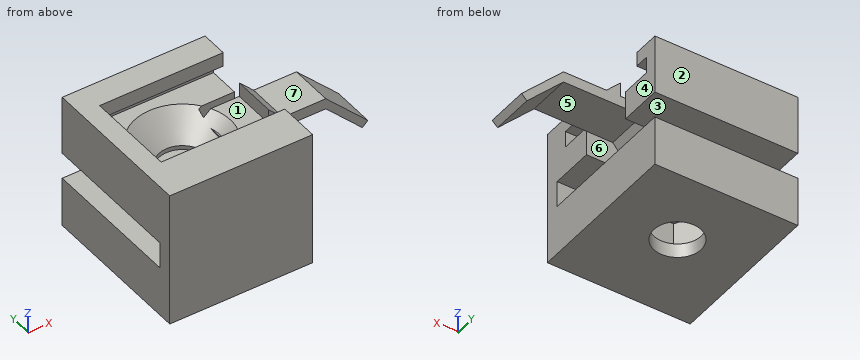
```python
from build123d import *

# Parameters (mm, degrees)
CROQUIS1_W               = 20
CROQUIS1_H               = 20
CROQUIS1_R               = 3.1
SALIENTE_EXTRUIR1_DEPTH  = 4
SALIENTE_EXTRUIR2_DEPTH  = 2.3
SALIENTE_EXTRUIR4_DEPTH  = 2
SALIENTE_EXTRUIR5_DEPTH  = 4
SALIENTE_EXTRUIR6_START  = -6
SALIENTE_EXTRUIR6_DEPTH  = 6
CROQUIS10_W              = 5
CROQUIS10_H              = 1
CORTAR_EXTRUIR2_DEPTH    = 4
CORTAR_EXTRUIR3_START    = -13
CROQUIS11_W              = 2.5
CROQUIS11_H              = 6
CORTAR_EXTRUIR3_DEPTH    = 13
SALIENTE_EXTRUIR7_START  = -6
SALIENTE_EXTRUIR7_DEPTH  = 6
CROQUIS14_W              = 20
CROQUIS14_H              = 19
SALIENTE_EXTRUIR8_DEPTH  = 2
CROQUIS15_W              = 20
CROQUIS15_H              = 7
SALIENTE_EXTRUIR9_DEPTH  = 20
CORTAR_EXTRUIR4_DEPTH    = 5
CROQUIS17_R              = 3.3
CORTAR_EXTRUIR5_DEPTH    = 2
SALIENTE_EXTRUIR10_START = -6
SALIENTE_EXTRUIR10_DEPTH = 6


with BuildPart() as part:
    # Croquis1 → Saliente-Extruir1 (new body)
    with BuildSketch(Plane.XY):
        Rectangle(CROQUIS1_W, CROQUIS1_H)
        Circle(CROQUIS1_R, mode=Mode.SUBTRACT)
    extrude(amount=SALIENTE_EXTRUIR1_DEPTH)

    # Croquis3 → Saliente-Extruir2 (add)
    with BuildSketch(Plane.XY.offset(4)):
        Polygon((10, 10), (-10, 10), (-10, -10), (10, -10), (10, -8.3), (-7.3, -8.3), (-7.3, 8.3), (10, 8.3), align=None)
    extrude(amount=SALIENTE_EXTRUIR2_DEPTH)

    # Croquis6 → Saliente-Extruir4 (add)
    with BuildSketch(Plane.XY.offset(6.3)):
        Polygon((10, 10), (10, 6.3), (-7.3, 6.3), (-7.3, -6.3), (10, -6.3), (10, -10), (-10, -10), (-10, 10), align=None)
    extrude(amount=SALIENTE_EXTRUIR4_DEPTH)

    # Croquis7 → Saliente-Extruir5 (add)
    with BuildSketch(Plane.XY.offset(4)):
        Polygon((10, 0), (10, 3), (18, 3), (18, 0), (18, -3), (10, -3), align=None)
    extrude(amount=-SALIENTE_EXTRUIR5_DEPTH)

    # Croquis9 → Saliente-Extruir6 (add)
    with BuildSketch(Plane.XZ.offset(3).offset(SALIENTE_EXTRUIR6_START)):
        Polygon((12, 4), (10, 6), (10, 4), align=None)
    extrude(amount=SALIENTE_EXTRUIR6_DEPTH)

    # Croquis10 → Cortar-Extruir2 (cut)
    with BuildSketch(Plane.XY.offset(4)):
        with Locations((7.5, 3.5)):
            Rectangle(CROQUIS10_W, CROQUIS10_H)
        with Locations((7.5, -3.5)):
            Rectangle(CROQUIS10_W, CROQUIS10_H)
    extrude(amount=-CORTAR_EXTRUIR2_DEPTH, mode=Mode.SUBTRACT)

    # Croquis11 → Cortar-Extruir3 (cut)
    with BuildSketch(Plane(origin=(18, 0, 0), x_dir=(0, 0, -1), z_dir=(1, 0, 0)).offset(CORTAR_EXTRUIR3_START)):
        with Locations((-1.25, 0)):
            Rectangle(CROQUIS11_W, CROQUIS11_H)
    extrude(amount=CORTAR_EXTRUIR3_DEPTH, mode=Mode.SUBTRACT)

    # Croquis12 → Saliente-Extruir7 (add)
    with BuildSketch(Plane(origin=(0, 3, 0), x_dir=(1, 0, 0), z_dir=(0, 1, 0)).offset(SALIENTE_EXTRUIR7_START)):
        Polygon((18, -2.5), (23.125934171, 2.625934171), (23.875934171, 1.875934171), (18, -4), align=None)
    extrude(amount=SALIENTE_EXTRUIR7_DEPTH)

    # Croquis13 → Refrentado para tornillo tapón con cabeza plana de clavija de M61 (revolve, cut)
    with BuildSketch(Plane(origin=(0, 0, 4), x_dir=(0, -1, 0), z_dir=(1, 0, 0))):
        Polygon((0, 0), (0, 6.625934171), (3.3, 6.625934171), (3.3, 3.42), (6.72, 0), align=None)
    revolve(axis=Axis((0, 0, 10.35), (0, 0, -1)), mode=Mode.SUBTRACT)

    # Croquis14 → Saliente-Extruir8 (add)
    with BuildSketch(Plane.XZ.offset(10)):
        with Locations((0, -1.2)):
            Rectangle(CROQUIS14_W, CROQUIS14_H)
    extrude(amount=SALIENTE_EXTRUIR8_DEPTH)

    # Croquis15 → Saliente-Extruir9 (add)
    with BuildSketch(Plane(origin=(0, -10, 0), x_dir=(1, 0, 0), z_dir=(0, 1, 0))):
        with Locations((0, 7.2)):
            Rectangle(CROQUIS15_W, CROQUIS15_H)
    extrude(amount=SALIENTE_EXTRUIR9_DEPTH)

    # Croquis16 → Cortar-Extruir4 (cut)
    with BuildSketch(Plane.XY.offset(-3.7)):
        Polygon((5.802370205, 0), (2.901185103, 5.025), (-2.901185103, 5.025), (-5.802370205, 0), (-2.901185103, -5.025), (2.901185103, -5.025), align=None)
    extrude(amount=-CORTAR_EXTRUIR4_DEPTH, mode=Mode.SUBTRACT)

    # Croquis17 → Cortar-Extruir5 (cut)
    with BuildSketch(Plane.XY.offset(-8.7)):
        Circle(CROQUIS17_R)
    extrude(amount=-CORTAR_EXTRUIR5_DEPTH, mode=Mode.SUBTRACT)

    # Croquis19 → Saliente-Extruir10 (add)
    with BuildSketch(Plane.XZ.offset(3).offset(SALIENTE_EXTRUIR10_START)):
        Polygon((5, 2.5), (7, 2.5), (5, 0), align=None)
    extrude(amount=SALIENTE_EXTRUIR10_DEPTH)


solid = part.part
```
Check sheet for the modelled part. Datum: model origin and axes. Units: mm. Face numbers are marked on the shaded views. A direction names the side the tool comes from. Give positions to 0.01 mm unless a question says otherwise; leave off trailing zeros. Loops run counter-clockwise (first coordinate to the right, second up) from the corner with the lowest first, then second, coordinate; pieces in that order, holes last. Notation, with made-up numbers: M -16.5,-14.5 L 5.5,-14.5 A35 cw 5.5,23.5 Z; hole C -7.75,29 d9. An arc over 180 degrees is marked long. Answer in a Markdown table with one row per item.
1) Cross-section at A-A (z = 1.5). Enter the section's corners in (x, y).
Solutions:
| item | result |
|---|---|
| outline | M -10,-12 L 10,-12 L 10,-4 L 5,-4 L 5,-3 L 6.2,-3 L 6.2,3 L 5,3 L 5,4 L 10,4 L 10,10 L -10,10 Z; M 19,-3 L 20.5,-3 L 20.5,3 L 19,3 Z; hole C 0,0 d8.44 |
2) Tool access check on the marked faces 4, 5, 6 and 7. Record the directions out of +Z, -Z, +X, -X, +Y, -Y that give a thin tool (end or side, any length) a straight path to the whole face; none if there is none.
Solutions:
| item | result |
|---|---|
| face 4 | +Z, -Z, +X, +Y |
| face 5 | none |
| face 6 | +Z, +X |
| face 7 | +Z, +X, +Y, -Y |
3) Cross-section at D-D (x = 0). Count the separate pieces of the cut face and the enclosed holes in it, plus the area to 3 significant figures.
Solutions:
| item | result |
|---|---|
| separate pieces | 3 |
| enclosed holes | 0 |
| area | 179 mm^2 |
4) Cross-section at B-B (x = 8). Enter the section's corners in (y, z).
Solutions:
| item | result |
|---|---|
| outline | M -12,-10.7 L 10,-10.7 L 10,-3.7 L -10,-3.7 L -10,0 L -4,0 L -4,4 L -8.3,4 L -8.3,6.3 L -6.3,6.3 L -6.3,8.3 L -12,8.3 Z; M -3,2.5 L 3,2.5 L 3,4 L -3,4 Z; M 4,0 L 10,0 L 10,8.3 L 6.3,8.3 L 6.3,6.3 L 8.3,6.3 L 8.3,4 L 4,4 Z |
5) Mould release check, pull along Y, two halves, no side actions. Record for the marked faces 1, 2 and 3: released by +Y, released by -Y, zero draft, split by the parting line, or undercut.
Solutions:
| item | result |
|---|---|
| face 1 | undercut |
| face 2 | released by +Y |
| face 3 | zero draft |
6) Cross-section at C-C (z = -0.75). Enter the section's corners in (x, y), plus the area to 3 significant figures.
Solutions:
| item | result |
|---|---|
| outline | M -10,-12 L 10,-12 L 10,-10 L -10,-10 Z; M 21.25,-3 L 22.75,-3 L 22.75,3 L 21.25,3 Z |
| area | 49.0 mm^2 |
7) Depth check by flat-ended pin: pin 1 (1.5 mm diameter, centred on y = -6.5, z = 4, fed in from +X); pin 2 (0.8 mm diameter, centred on y = 3.5, z = 2, fed in from +X); pin 3 (4 mm diameter, centred on y = -2, z = -0.5, fed in from -X); pin 4 (1.2 mm diameter, centred on x = 7.5, y = 1.5, fed in from +Z). Enter the tip coordinate at first touch or a pass-through.
Solutions:
| item | result |
|---|---|
| pin 1 | stops at x = 10 |
| pin 2 | stops at x = 5 |
| pin 3 | stops at x = -10 |
| pin 4 | stops at z = 4 |
8) Thickness scan on line 1 (Z direction, x = -7, y = -8.25); line 2 (Z direction, x = -8, y = 6.5); line 3 (Y direction, x = 0, z = -10.1). Record the ranges inside material, lowest first.
Solutions:
| item | result |
|---|---|
| line 1 | z = -10.7 to -3.7, 0 to 4, 6.3 to 8.3 |
| line 2 | z = -10.7 to -3.7, 0 to 8.3 |
| line 3 | y = -12 to -3.3, 3.3 to 10 |
